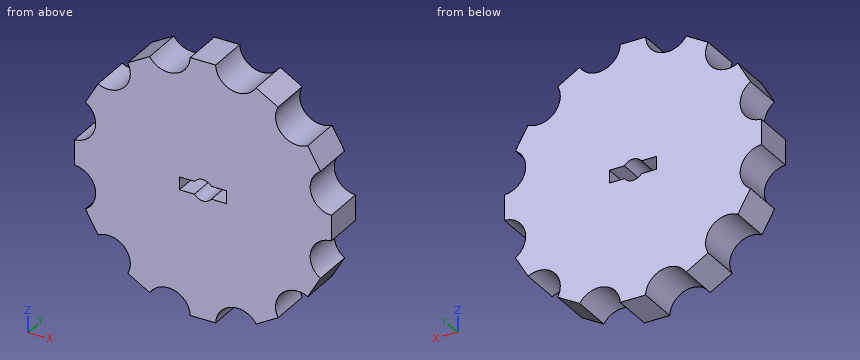
from build123d import *

# Parameters (mm, degrees)
BOSS_EXTRUDE1_DEPTH = 9.6
CUT_EXTRUDE1_DEPTH  = 44.617034843


with BuildPart() as part:
    # Sketch1 → Boss-Extrude1 (new body)
    with BuildSketch(Plane(origin=(0, 0, 0), x_dir=(1, 0, 0), z_dir=(0, 1, 0))):
        with BuildLine():
            ThreePointArc((-12.471666355, -27.539329703), (-6.782081918, -25.311074298), (-2.96888496, -30.085592303))
            Line((-2.96888496, -30.085592303), (2.96888496, -30.085592303))
            ThreePointArc((2.96888496, -30.085592303), (6.782081918, -25.311074298), (12.471666355, -27.539329703))
            Line((12.471666355, -27.539329703), (17.613925948, -24.570444742))
            ThreePointArc((17.613925948, -24.570444742), (18.52899238, -18.52899238), (24.570444742, -17.613925948))
            Line((24.570444742, -17.613925948), (27.539329703, -12.471666355))
            ThreePointArc((27.539329703, -12.471666355), (25.311074298, -6.782081918), (30.085592303, -2.96888496))
            Line((30.085592303, -2.96888496), (30.085592303, 2.96888496))
            ThreePointArc((30.085592303, 2.96888496), (25.311074298, 6.782081918), (27.539329703, 12.471666355))
            Line((27.539329703, 12.471666355), (24.570444742, 17.613925948))
            ThreePointArc((24.570444742, 17.613925948), (18.52899238, 18.52899238), (17.613925948, 24.570444742))
            Line((17.613925948, 24.570444742), (12.471666355, 27.539329703))
            ThreePointArc((12.471666355, 27.539329703), (6.782081918, 25.311074298), (2.96888496, 30.085592303))
            Line((2.96888496, 30.085592303), (-2.96888496, 30.085592303))
            ThreePointArc((-2.96888496, 30.085592303), (-6.782081918, 25.311074298), (-12.471666355, 27.539329703))
            Line((-12.471666355, 27.539329703), (-17.613925948, 24.570444742))
            ThreePointArc((-17.613925948, 24.570444742), (-18.52899238, 18.52899238), (-24.570444742, 17.613925948))
            Line((-24.570444742, 17.613925948), (-27.539329703, 12.471666355))
            ThreePointArc((-27.539329703, 12.471666355), (-25.311074298, 6.782081918), (-30.085592303, 2.96888496))
            Line((-30.085592303, 2.96888496), (-30.085592303, -2.96888496))
            ThreePointArc((-30.085592303, -2.96888496), (-25.311074298, -6.782081918), (-27.539329703, -12.471666355))
            Line((-27.539329703, -12.471666355), (-24.570444742, -17.613925948))
            ThreePointArc((-24.570444742, -17.613925948), (-18.52899238, -18.52899238), (-17.613925948, -24.570444742))
            Line((-17.613925948, -24.570444742), (-12.471666355, -27.539329703))
        make_face()
    extrude(amount=BOSS_EXTRUDE1_DEPTH)

    # Sketch2 → Cut-Extrude1 (cut, through all)
    with BuildSketch(Plane(origin=(0, 9.6, 0), x_dir=(1, 0, 0), z_dir=(0, 1, 0))):
        with BuildLine():
            Line((-2, -1.5), (-5.5, -1.5))
            Line((-5.5, -1.5), (-5.5, 1.5))
            Line((-5.5, 1.5), (-2, 1.5))
            ThreePointArc((-2, 1.5), (0, 2.5), (2, 1.5))
            Line((2, 1.5), (5.5, 1.5))
            Line((5.5, 1.5), (5.5, -1.5))
            Line((5.5, -1.5), (2, -1.5))
            ThreePointArc((2, -1.5), (0, -2.5), (-2, -1.5))
        make_face()
    extrude(amount=-CUT_EXTRUDE1_DEPTH, mode=Mode.SUBTRACT)


solid = part.part
Design review of the part built by this model. Coordinates are the model's own, in mm. Give positions to 0.01 mm unless a question says otherwise; leave off trailing zeros. Loops run counter-clockwise (first coordinate to the right, second up) from the corner with the lowest first, then second, coordinate; pieces in that order, holes last. Notation, with made-up numbers: M -28,52.5 L -18,52.5 A24 ccw -18,69.5 Z; hole C 28.5,47 d6. An arc over 180 degrees is marked long. Write item = value, one per line.
Q1. We need section B-B (z = -21). Give the boundary of the cut face in (x, y), plus the area to 3 significant figures.
Output values:
outline = M -17.16,0 L 17.16,0 L 17.16,9.6 L -17.16,9.6 Z
area = 329 mm^2
Q2. To check wall thickness, follow line 1 (Z direction, x = 12.5, y = 4); line 2 (Z direction, x = -26.5, y = 1.75); line 3 (X direction, y = 4.25, z = -23). State the ranges of each line that lie inside material, in increasing order. Write a range as [from, to].
Output values:
line_1 = [-27.52, 27.52]
line_2 = [-14.27, -11.61], [-4.62, 4.62], [11.61, 14.27]
line_3 = [-17.09, 17.09]
Q3. Insertion check: pin 1 (4 mm diameter, centred on x = -11.5, y = 2, fed in from +Z); pin 2 (5 mm diameter, centred on x = -22, y = 3, fed in from +Z); pin 3 (1.5 mm diameter, centred on x = -7, y = 8, fed in from -Z). Each pin has a flat end and moves straight along its axis. Give the tip position at first contact, or say it passes through.
Output values:
pin_1 = 27.54
pin_2 = 17.77
pin_3 = -25.49
Q4. We need section C-C (x = 19). Give the boundary of the cut face in (y, z).
Output values:
outline = M 0,-18.11 L 9.6,-18.11 L 9.6,18.11 L 0,18.11 Z
